Source: CAD feature listing. Evaluate the final solid. Frame: model axes, mm. A direction names the side the tool comes from. Give positions to 0.01 mm unless a question says otherwise; leave off trailing zeros. Order: outer loops, then holes, each group sorted by start corner. A loop starts at its lowest first (then second) coordinate and runs counter-clockwise, first axis right, second up.
```python
from build123d import *

# Parameters (mm, degrees)
SKETCH1_R           = 30
SKETCH1_R_2         = 25
BOSS_EXTRUDE1_DEPTH = 10
SKETCH3_R           = 5
BOSS_EXTRUDE2_DEPTH = 5
CUT_EXTRUDE1_DEPTH  = 5
FILLET3_R           = 5
FILLET4_R           = 5
FILLET5_R           = 5
FILLET6_R           = 5
FILLET7_R           = 5
FILLET8_R           = 5


with BuildPart() as part:
    # Sketch1 → Boss-Extrude1 (new, symmetric)
    with BuildSketch(Plane(origin=(0, 0, 0), x_dir=(1, 0, 0), z_dir=(0, 1, 0))):
        with Locations(Location((0, 0, 0), (0, 0, 270))):
            Circle(SKETCH1_R)
        with Locations(Location((0, 0, 0), (0, 0, 270))):
            Circle(SKETCH1_R_2, mode=Mode.SUBTRACT)
    extrude(amount=BOSS_EXTRUDE1_DEPTH, both=True)

    # Sketch3 → Boss-Extrude2 (add)
    # profile 1 of 3: a face of its own
    with BuildSketch(Plane(origin=(0, 10, 0), x_dir=(1, 0, 0), z_dir=(0, 1, 0))):
        with BuildLine():
            Line((-39.570552361, 7.72740661), (-27.975291142, 10.83434749))
            ThreePointArc((-27.975291142, 10.83434749), (-30, 0), (-27.975291142, -10.83434749))
            Line((-27.975291142, -10.83434749), (-39.570552361, -7.72740661))
            ThreePointArc((-39.570552361, -7.72740661), (-45.5, 0), (-39.570552361, 7.72740661))
        make_face()
        with Locations(Location((-37.5, 0, 0), (0, 0, 270))):
            Circle(SKETCH3_R, mode=Mode.SUBTRACT)
    # profile 2 of 3: a face of its own
    with BuildSketch(Plane(origin=(0, 10, 0), x_dir=(1, 0, 0), z_dir=(0, 1, 0))):
        with BuildLine():
            Line((26.47740661, 30.405400281), (23.370465731, 18.810139062))
            ThreePointArc((23.370465731, 18.810139062), (15, 25.980762114), (4.604825411, 29.644486552))
            Line((4.604825411, 29.644486552), (13.093145751, 38.132806891))
            ThreePointArc((13.093145751, 38.132806891), (22.75, 39.404155872), (26.47740661, 30.405400281))
        make_face()
        with Locations(Location((18.75, 32.475952642, 0), (0, 0, 270))):
            Circle(SKETCH3_R, mode=Mode.SUBTRACT)
    # profile 3 of 3: a face of its own
    with BuildSketch(Plane(origin=(0, 10, 0), x_dir=(1, 0, 0), z_dir=(0, 1, 0))):
        with BuildLine():
            Line((13.093145751, -38.132806891), (4.604825411, -29.644486552))
            ThreePointArc((4.604825411, -29.644486552), (15, -25.980762114), (23.370465731, -18.810139062))
            Line((23.370465731, -18.810139062), (26.47740661, -30.405400281))
            ThreePointArc((26.47740661, -30.405400281), (22.75, -39.404155872), (13.093145751, -38.132806891))
        make_face()
        with Locations(Location((18.75, -32.475952642, 0), (0, 0, 270))):
            Circle(SKETCH3_R, mode=Mode.SUBTRACT)
    boss_extrude2 = extrude(amount=-BOSS_EXTRUDE2_DEPTH)

    # Mirror1: Boss-Extrude2 across plane
    add(boss_extrude2.mirror(Plane.ZX))

    # Sketch4 → Cut-Extrude1 (cut, symmetric)
    with BuildSketch(Plane(origin=(0, 0, 0), x_dir=(1, 0, 0), z_dir=(0, 1, 0))):
        with BuildLine():
            ThreePointArc((-17.67766953, 17.67766953), (-25, 0), (-17.67766953, -17.67766953))
            Line((-17.67766953, -17.67766953), (-21.213203436, -21.213203436))
            ThreePointArc((-21.213203436, -21.213203436), (-30, 0), (-21.213203436, 21.213203436))
            Line((-21.213203436, 21.213203436), (-17.67766953, 17.67766953))
        make_face()
        with BuildLine():
            Line((24.148145657, -6.470476128), (28.977774789, -7.764571353))
            ThreePointArc((28.977774789, -7.764571353), (15, -25.980762114), (-7.764571353, -28.977774789))
            Line((-7.764571353, -28.977774789), (-6.470476128, -24.148145657))
            ThreePointArc((-6.470476128, -24.148145657), (12.5, -21.650635095), (24.148145657, -6.470476128))
        make_face()
        with BuildLine():
            Line((-6.470476128, 24.148145657), (-7.764571353, 28.977774789))
            ThreePointArc((-7.764571353, 28.977774789), (15, 25.980762114), (28.977774789, 7.764571353))
            Line((28.977774789, 7.764571353), (24.148145657, 6.470476128))
            ThreePointArc((24.148145657, 6.470476128), (12.5, 21.650635095), (-6.470476128, 24.148145657))
        make_face()
    extrude(amount=CUT_EXTRUDE1_DEPTH, both=True, mode=Mode.SUBTRACT)

    # Fillet3
    fillet3_edges = [part.edges().sort_by_distance(p)[0] for p in [
        (-19.445436483, -5, -19.445436483),
        (-19.445436483, 5, -19.445436483),
    ]]
    fillet(fillet3_edges, radius=FILLET3_R - 0.0001)  # a hair under: the kernel refuses the full size

    # Fillet4
    fillet4_edges = [part.edges().sort_by_distance(p)[0] for p in [
        (-19.445436483, 5, 19.445436483),
        (-19.445436483, -5, 19.445436483),
    ]]
    fillet(fillet4_edges, radius=FILLET4_R - 0.0001)  # a hair under: the kernel refuses the full size

    # Fillet5
    fillet5_edges = [part.edges().sort_by_distance(p)[0] for p in [
        (-7.11752374, -5, 26.562960223),
        (-7.11752374, 5, 26.562960223),
    ]]
    fillet(fillet5_edges, radius=FILLET5_R - 0.0001)  # a hair under: the kernel refuses the full size

    # Fillet6
    fillet6_edges = [part.edges().sort_by_distance(p)[0] for p in [
        (26.562960223, 5, 7.11752374),
        (26.562960223, -5, 7.11752374),
    ]]
    fillet(fillet6_edges, radius=FILLET6_R - 0.0001)  # a hair under: the kernel refuses the full size

    # Fillet7
    fillet7_edges = [part.edges().sort_by_distance(p)[0] for p in [
        (26.562960223, -5, -7.11752374),
        (26.562960223, 5, -7.11752374),
    ]]
    fillet(fillet7_edges, radius=FILLET7_R - 0.0001)  # a hair under: the kernel refuses the full size

    # Fillet8
    fillet8_edges = [part.edges().sort_by_distance(p)[0] for p in [
        (-7.11752374, 5, -26.562960223),
        (-7.11752374, -5, -26.562960223),
    ]]
    fillet(fillet8_edges, radius=FILLET8_R - 0.0001)  # a hair under: the kernel refuses the full size


solid = part.part
```
1) Section query C-C, the plane x = 0. Return the cut outline in (y, z).
Report:
outline: (-10, -30) - (-5, -30) - (-5, -25) - (-10, -25) - close; (-10, 25) - (-5, 25) - (-5, 30) - (-10, 30) - close; (5, -30) - (10, -30) - (10, -25) - (5, -25) - close; (5, 25) - (10, 25) - (10, 30) - (5, 30) - close
2) Section query D-D, the plane x = 15.5. Count the separate pieces of the cut face and the enclosed holes in it, and give its area (3 significant figures).
Report:
separate pieces: 8
enclosed holes: 0
area: 251 mm2
3) Material intervals for L1, parallel to Y at x = -25, z = -8.5; L2, parallel to X at y = -7.15, z = 0; L3, parallel to Z at x = 22, y = 7, sorted ascending.
Report:
L1: y = -10 to -5, 5 to 10
L2: x = -45.5 to -42.5, -32.5 to -25, 25 to 30
L3: z = -39.79 to -36.28, -28.68 to -11.87, 11.87 to 28.68, 36.28 to 39.79
4) Section query B-B, the plane z = 0. Return the cut outline in (x, y), and give its area (3 significant figures).
Report:
outline: (-45.5, -10) - (-42.5, -10) - (-42.5, -5) - (-45.5, -5) - close; (-45.5, 5) - (-42.5, 5) - (-42.5, 10) - (-45.5, 10) - close; (-32.5, -10) - (-25, -10) - (-25, -5) - (-32.5, -5) - close; (-32.5, 5) - (-25, 5) - (-25, 10) - (-32.5, 10) - close; (25, -10) - (30, -10) - (30, 10) - (25, 10) - close
area: 205 mm2
5) Section query A-A, the plane y = -6.25. Return the cut outline in (x, z).
Report:
outline: (-39.57, -7.73) - (-27.98, -10.83) arc R30 ccw to (4.6, -29.64) - (13.09, -38.13) arc R8 ccw to (26.48, -30.41) - (23.37, -18.81) arc R30 ccw to (23.37, 18.81) - (26.48, 30.41) arc R8 ccw to (13.09, 38.13) - (4.6, 29.64) arc R30 ccw to (-27.98, 10.83) - (-39.57, 7.73) arc R8 ccw to start; hole circle Ø10 at (-37.5, 0); hole circle Ø50 at (0, 0); hole circle Ø10 at (18.75, -32.48); hole circle Ø10 at (18.75, 32.48)
6) Draft query along Z for faces 1 (the cylindrical face through (25.97, -3.57, 8.51)), 2 (the flat face through (-33.85, -7.54, -9.26)), 3 (the cylindrical face through (-32.543, -7.535, -0.651)). Return one class per face: +Z half, -Z half, draft (parallel to the pull), parting line (faces both ways), or undercut.
Report:
face 1: +Z half
face 2: -Z half
face 3: undercut
7) Reachability of faces 4 (the cylindrical face through (-5.59, 3.574, 26.671)), 5 (the cylindrical face through (-20.302, 3.496, 18.286)), 6 (the cylindrical face through (-5.68, 3.5, -26.73)) from +Z, -Z, +X, -X, +Y, -Y: full face, straight path, thin tool, end or side. Return the list, or none.
Report:
face 4: +Z, +X
face 5: -X
face 6: -Z, +X
8) Pin query (flat end, axial travel): pin 1 (2 mm diameter, centred on x = -28, y = -7.5, fed in from -Z); pin 2 (6 mm diameter, centred on x = -37.5, z = 0, fed in from +Y); pin 3 (5 mm diameter, centred on y = -2.5, z = -5.5, fed in from +X); pin 4 (5 mm diameter, centred on y = -1, z = -26, fed in from +X). Return the tip coordinate at first contact, or that it passes through.
Report:
pin 1: stops at z = -13.08
pin 2: passes through
pin 3: stops at x = 29.85
pin 4: stops at x = -5.4
